Check sheet for the drawn part. Datum: minimum x, y, z corner. Units: mm. Round coordinates to 2 decimals unless told otherwise and drop trailing zeros. Order: outer loops, then holes, each group sorted by start corner. A loop starts at its lowest first (then second) coordinate and runs counter-clockwise, first axis right, second up. Notation, with made-up numbers: (1.25, 34.25) -> (16.25, 34.25) arc R14 ccw to (16.25, 56.25) -> close; hole circle Ø6 at (47, 0.5). An arc over 180 degrees is marked (long way). Answer in a Markdown table with one row per item.
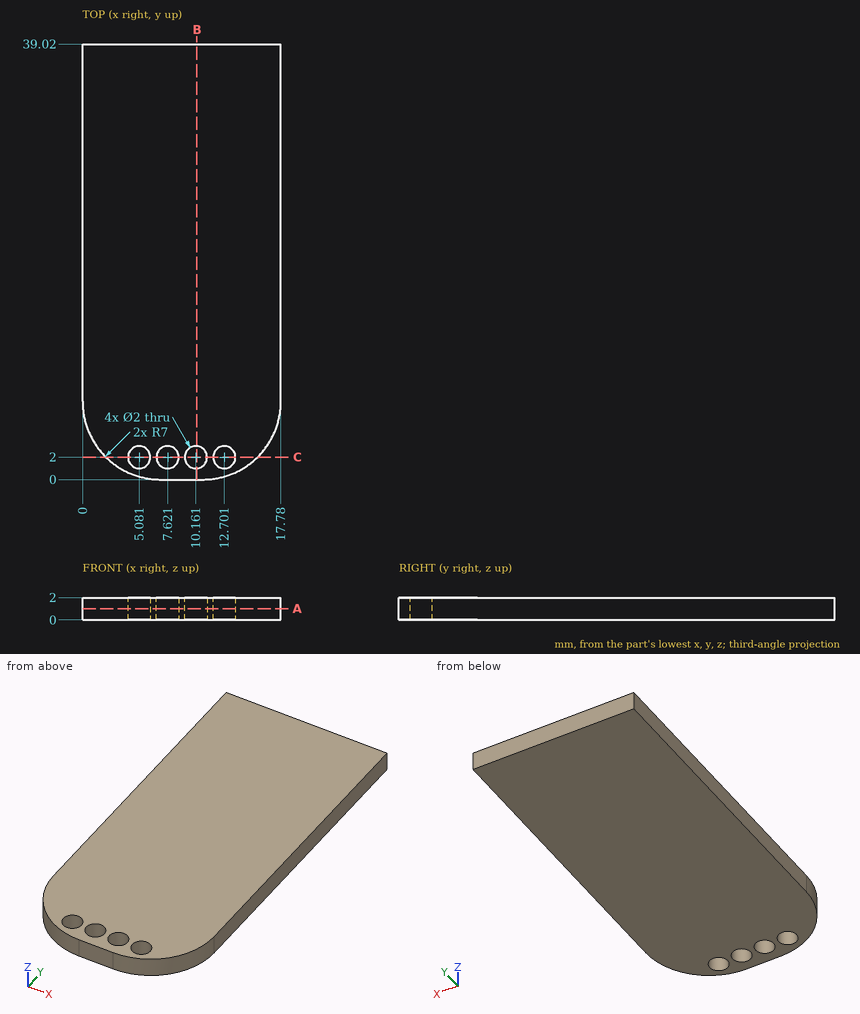
(1) Section check A-A on z = 1. Record the boundary of the cut face in (x, y), plus the area to 3 significant figures.
Solutions:
| item | result |
|---|---|
| outline | (0, 7) arc R7 ccw to (7, 0) -> (10.78, 0) arc R7 ccw to (17.78, 7) -> (17.78, 39.02) -> (0, 39.02) -> close; hole circle Ø2 at (5.08, 2); hole circle Ø2 at (7.62, 2); hole circle Ø2 at (10.16, 2); hole circle Ø2 at (12.7, 2) |
| area | 660 mm^2 |
(2) Scan lines: probe 1 along Y at (x, z) = (12.25, 1.5) (1 decimal); probe 2 along Y at (x, z) = (14.75, 1.8) (1 decimal); probe 3 along Y at (x, z) = (16.75, 0.9) (1 decimal). Record each from-to range of solid material in increasing order. Write a range as from..to.
Solutions:
| item | result |
|---|---|
| probe 1 | 0.2..1.1, 2.9..39 |
| probe 2 | 1.2..39 |
| probe 3 | 3.3..39 |
(3) Section check B-B on x = 10.25. Record the boundary of the cut face in (y, z).
Solutions:
| item | result |
|---|---|
| outline | (0, 0) -> (1, 0) -> (1, 2) -> (0, 2) -> close; (3, 0) -> (39.02, 0) -> (39.02, 2) -> (3, 2) -> close |
(4) Section check C-C on y = 2. Record the boundary of the cut face in (x, z).
Solutions:
| item | result |
|---|---|
| outline | (2.1, 0) -> (4.08, 0) -> (4.08, 2) -> (2.1, 2) -> close; (6.08, 0) -> (6.62, 0) -> (6.62, 2) -> (6.08, 2) -> close; (8.62, 0) -> (9.16, 0) -> (9.16, 2) -> (8.62, 2) -> close; (11.16, 0) -> (11.7, 0) -> (11.7, 2) -> (11.16, 2) -> close; (13.7, 0) -> (15.68, 0) -> (15.68, 2) -> (13.7, 2) -> close |
(5) Depth check by flat-ended pin: pin 1 Ø1.6 at (x, y) = (7.62, 2) entering from -Z. Enter the tip coordinate at first touch or a pass-through.
Solutions:
| item | result |
|---|---|
| pin 1 | through |
